from build123d import *

# Parameters (mm, degrees)
SALIENTE_EXTRUIR1_DEPTH = 8
REDONDEO1_R             = 5
REDONDEO2_R             = 5
REDONDEO3_R             = 1
CROQUIS2_R              = 3.6
CORTAR_EXTRUIR1_DEPTH   = 2


with BuildPart() as part:
    # Croquis1 → Saliente-Extruir1 (new body)
    with BuildSketch(Plane.XY):
        with BuildLine():
            Line((69, -45), (70, -45))
            ThreePointArc((70, -45), (73.535533906, -43.535533906), (75, -40))
            Line((75, -40), (75, 30))
            ThreePointArc((75, 30), (70.606601718, 40.606601718), (60, 45))
            Line((60, 45), (-60, 45))
            ThreePointArc((-60, 45), (-70.606601718, 40.606601718), (-75, 30))
            Line((-75, 30), (-75, -40))
            ThreePointArc((-75, -40), (-73.535533906, -43.535533906), (-70, -45))
            Line((-70, -45), (-69, -45))
            Line((-69, -45), (-69, -27.7))
            Line((-69, -27.7), (-31, -27.7))
            Line((-31, -27.7), (-31, -45))
            Line((-31, -45), (46, -45))
            Line((46, -45), (46, -27.7))
            Line((46, -27.7), (69, -27.7))
            Line((69, -27.7), (69, -45))
        make_face()
    extrude(amount=SALIENTE_EXTRUIR1_DEPTH)

    # Redondeo1
    redondeo1_edges = [part.edges().sort_by_distance(p)[0] for p in [
        (73.535533906, -43.535533906, 8),
        (75, -5, 8),
        (70.606601718, 40.606601718, 8),
        (0, 45, 8),
        (-70.606601718, 40.606601718, 8),
        (-75, -5, 8),
        (-73.535533906, -43.535533906, 8),
        (-69.5, -45, 8),
        (69.5, -45, 8),
    ]]
    fillet(redondeo1_edges, radius=REDONDEO1_R)

    # Redondeo2
    redondeo2_edges = [part.edges().sort_by_distance(p)[0] for p in [
        (7.5, -45, 8),
    ]]
    fillet(redondeo2_edges, radius=REDONDEO2_R)

    # Redondeo3
    redondeo3_edges = [part.edges().sort_by_distance(p)[0] for p in [
        (-69, -33.85, 8),
        (-50, -27.7, 8),
        (69, -33.85, 8),
        (69, -45, 1.5),
        (69, -43.535533906, 6.535533906),
        (-31, -33.85, 8),
        (-69, -45, 1.5),
        (-69, -43.535533906, 6.535533906),
        (57.5, -27.7, 8),
        (46, -33.85, 8),
        (46, -45, 1.5),
        (-31, -45, 1.5),
        (-31, -43.535533906, 6.535533906),
        (46, -43.535533906, 6.535533906),
    ]]
    fillet(redondeo3_edges, radius=REDONDEO3_R - 0.0001)  # a hair under: the kernel refuses the full size

    # Croquis2 → Cortar-Extruir1 (cut)
    with BuildSketch(Plane(origin=(0, 0, 0), x_dir=(-1, 0, 0), z_dir=(0, 0, -1))):
        with Locations((67, -19.7)):
            Circle(CROQUIS2_R)
        with Locations((64.071067812, 34.071067812)):
            Circle(CROQUIS2_R)
        with Locations((-67, -19.7)):
            Circle(CROQUIS2_R)
        with Locations((-64.071067812, 34.071067812)):
            Circle(CROQUIS2_R)
    extrude(amount=-CORTAR_EXTRUIR1_DEPTH, mode=Mode.SUBTRACT)


solid = part.part
Could you check a few things on this model? Use its own coordinates, in mm. A direction names the side the tool comes from. Give positions to 0.01 mm unless a question says otherwise; leave off trailing zeros. Order: outer loops, then holes, each group sorted by start corner. A loop starts at its lowest first (then second) coordinate and runs counter-clockwise, first axis right, second up.
Item 1: I need wall thicknesses on line 1 (X direction, y = -29, z = 1); line 2 (Y direction, x = 67, z = 1.6); line 3 (X direction, y = -34.5, z = 6). Which ranges of each line are inside material? Lowest first, please.
Item 2: If we section it at B-B, the plane x = 51.5: Write out the boundary of the cut face in (y, z), plus the area to 3 significant figures.
Item 3: For faces 1 (the face through (-67, -20, 2)), 2 (the face through (-1, 11, 0)), 3 (the face through (46, -36, 3)), which set-ups out of +Z, -Z, +X, -X, +Y, -Y let a thin tool reach every point of the face, with its end or its side?
Item 4: If we section it at A-A, the plane y = -35: Count the separate pieces of the cut face and the enclosed holes in it, plus the area to 3 significant figures.
Item 5: If we mould it in two halves opening along Y, with no side actions, what happens to faces 4 (the face through (67.668, 34.229, 0.986)), 5 (the face through (-1, 44, 6)), 6 (the face through (67, -20, 2)), 7 (the face through (74, -5, 6))? For each: pulls with the +Y half, pulls with the -Y half, needs draft (parallel to the pull), parting line crosses it, or undercut.
Item 6: If we section it at C-C, the plane y = -19.7: Write out the boundary of the cut face in (x, z), plus the area to 3 significant figures.
Item 7: I'm going to push flat-ended pins straight in: pin 1 (3.5 mm diameter, centred on y = -33.5, z = 3.5, fed in from +X); pin 2 (2 mm diameter, centred on x = 67.5, y = -18, fed in from -Z); pin 3 (2 mm diameter, centred on x = 52, z = 3, fed in from -Y); pin 4 (3 mm diameter, centred on y = -15.5, z = 6, fed in from +X). Where does each tip first touch, or does it pass through?
Values:
1. line 1: x = -75 to -69, -31 to 46, 69 to 75
1. line 2: y = -27.7 to -23.3, -16.1 to 31.98, 36.16 to 43.27
1. line 3: x = -74 to -69, -31 to 46, 69 to 74
2. outline: (-27.7, 0) - (45, 0) - (45, 3) arc R5 ccw to (40, 8) - (-26.7, 8) arc R1 ccw to (-27.7, 7) - close
2. area: 576 mm2
3. face 1: -Z
3. face 2: -Z, +X, -X, +Y, -Y
3. face 3: +Z, -Z, -Y
4. separate pieces: 3
4. enclosed holes: 0
4. area: 700 mm2
5. face 4: undercut
5. face 5: pulls with the +Y half
5. face 6: undercut
5. face 7: needs draft
6. outline: (-75, 0) - (-70.6, 0) - (-70.6, 2) - (-63.4, 2) - (-63.4, 0) - (63.4, 0) - (63.4, 2) - (70.6, 2) - (70.6, 0) - (75, 0) - (75, 3) arc R5 ccw to (70, 8) - (-70, 8) arc R5 ccw to (-75, 3) - close
6. area: 1,160 mm2
7. pin 1: stops at x = 75
7. pin 2: stops at z = 2
7. pin 3: stops at y = -27.7
7. pin 4: stops at x = 74.77
